from build123d import *

# Parameters (mm, degrees)
F0_W     = 533.4
F0_H     = 317.5
F1_DEPTH = 53.975
F2_W     = 533.4
F2_H     = 53.975
F3_DEPTH = 317.5


with BuildPart() as f1:
    # F0 (on Top) → F1 (new body, symmetric)
    with BuildSketch(Plane.XY):
        Rectangle(F0_W, F0_H)
    extrude(amount=F1_DEPTH, both=True)

    # F2 (on Top) → F3 (join)
    with BuildSketch(Plane.XY):
        with Locations((0, 185.7375)):
            Rectangle(F2_W, F2_H)
    extrude(amount=F3_DEPTH)


solid = f1.part
Geometry: final body of the model. Coordinates: model frame, mm. A direction names the side the tool comes from. Give positions to 0.01 mm unless a question says otherwise; leave off trailing zeros. Loops run counter-clockwise (first coordinate to the right, second up) from the corner with the lowest first, then second, coordinate; pieces in that order, holes last. Notation, with made-up numbers: (12.25, 50) - (57.25, 50) arc R22 cw to (57.25, 86) - close; hole circle Ø5 at (-25, 76). An arc over 180 degrees is marked (long way). One line per question, with ' | ' between items. Start each with the question number.
(1) Section query A-A on x = -144. Return loops of the section in (y, z) (3 decimals), then the cut area to 3 significant figures.
(2) Section query B-B on z = 99. Return loops of the section in (x, y) (3 decimals), then the cut area to 3 significant figures.
(3) Ray query, line 1 (Y direction, x = 64, z = 108) (3 decimals); line 2 (Z direction, x = 163.5, y = 189); line 3 (Z direction, x = -4, y = -128) (3 decimals). Return the intervals inside material, ascending. Write a range as from..to.
(4) Reachability of faces 1 (the flat face through (-4, 2, 53.975)), 2 (the flat face through (-4, 158.75, -27)), 3 (the flat face through (-4, 212.725, 157)) from +Z, -Z, +X, -X, +Y, -Y: full face, straight path, thin tool, end or side. Return the list, or none.
(5) Contact query for flat-ended pins moving along their axis: pin 1 (4 mm diameter, centred on x = -92.5, z = 268, fed in from -Y); pin 2 (6 mm diameter, centred on x = 16, y = 85, fed in from +Z) (3 decimals); pin 3 (16 mm diameter, centred on x = -11.5, z = -15, fed in from +Y). Output: stop coordinate, or through.
(6) Section query C-C on y = -62. Return loops of the section in (x, z) (3 decimals).
The answers:
1) outline: (-158.75, -53.975) - (158.75, -53.975) - (158.75, 0) - (212.725, 0) - (212.725, 317.5) - (158.75, 317.5) - (158.75, 53.975) - (-158.75, 53.975) - close | area: 51,400 mm2
2) outline: (-266.7, 158.75) - (266.7, 158.75) - (266.7, 212.725) - (-266.7, 212.725) - close | area: 28,800 mm2
3) line 1: 158.75..212.725 | line 2: 0..317.5 | line 3: -53.975..53.975
4) face 1: +Z, +X, -X, -Y | face 2: -Z, +X, -X, +Y | face 3: +Z, -Z, +X, -X, +Y
5) pin 1: y = 158.75 | pin 2: z = 53.975 | pin 3: y = 158.75
6) outline: (-266.7, -53.975) - (266.7, -53.975) - (266.7, 53.975) - (-266.7, 53.975) - close
